Part print with two shaded views. Sizes in mm from the minimum x, y, z corner. A direction names the side the tool comes from. Coordinates: 2 decimals unless noted, no trailing zeros. Loops run counter-clockwise (first coordinate to the right, second up) from the corner with the lowest first, then second, coordinate; pieces in that order, holes last.
(1) Wall check: L1, parallel to Y at x = 14, z = 1.5; L2, parallel to Y at x = 14, z = 6.75; L3, parallel to X at y = 18, z = 1.5 (1 decimal). Give the ranges that are in metal, low to high.
(2) Slice it at C-C (z = 1). Give the cut face in (x, y).
(3) Two-plate mould, pull along Y, no slides. Class the marked faces 1, 2 and 3: pulls with the +Y half, pulls with the -Y half, needs draft (parallel to the pull), parting line crosses it, or undercut.
(4) Slice it at B-B (y = 14). Give the cut face in (x, z), and give its area (3 significant figures).
(5) Tool access for the marked faces 4 and 5: list every direction of +Z, -Z, +X, -X, +Y, -Y with a clear straight run to the whole face (end or side of a thin tool).
(6) Flat gauge pins, fed straight in: P1, Ø1.5, axis at y = 15.5, z = 5, coming from the +X side; P2, Ø2.5, axis at x = 23.09, y = 8.75, coming from the +Z side; P3, Ø8, axis at x = 14, y = 14, coming from the +Z side; P4, Ø1.5, axis at y = 10.5, z = 7.5, coming from the +X side. Where does each tip first touch, or does it go through?
(7) Slice it at D-D (z = 8.5). Give the cut face in (x, y), and give its area (3 significant figures).
(8) Slice it at A-A (x = 14). Give the cut face in (y, z).
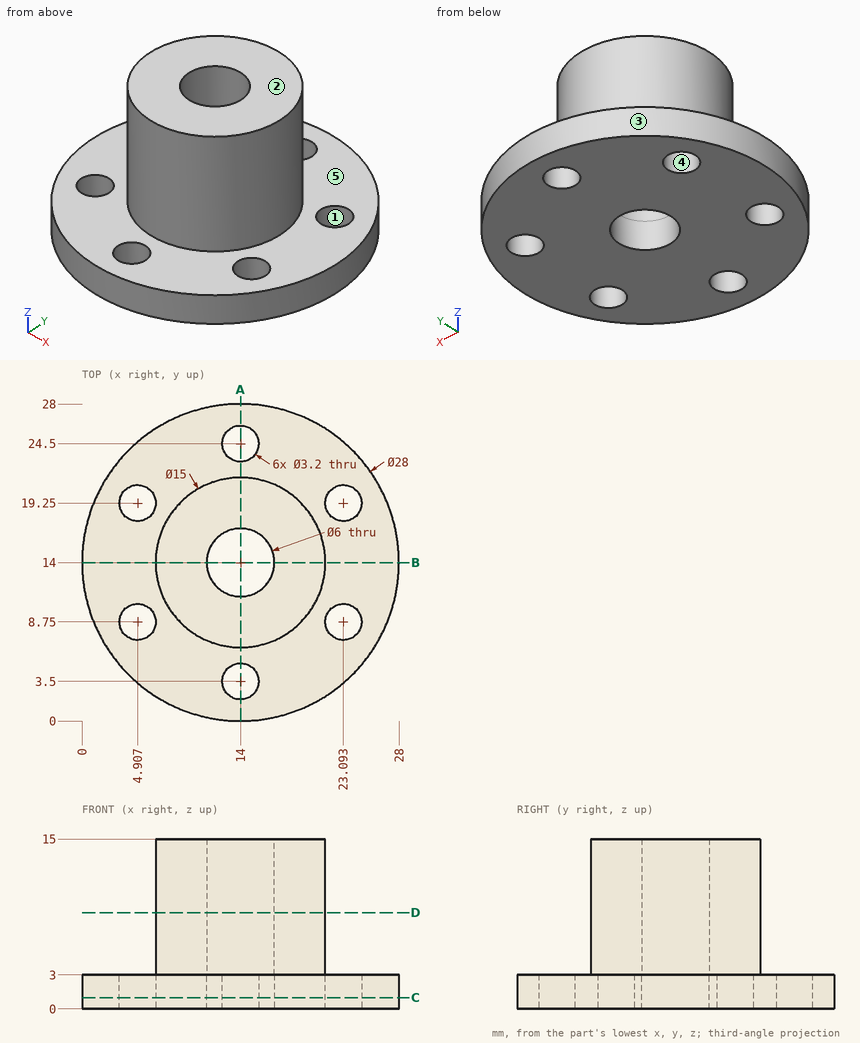
Response values:
1. L1: y = 0 to 1.9, 5.1 to 11, 17 to 22.9, 26.1 to 28
1. L2: y = 6.5 to 11, 17 to 21.5
1. L3: x = 0.6 to 3.9, 5.9 to 22.1, 24.1 to 27.4
2. outline: circle Ø28 at (14, 14); hole circle Ø3.2 at (4.91, 8.75); hole circle Ø3.2 at (4.91, 19.25); hole circle Ø6 at (14, 14); hole circle Ø3.2 at (14, 3.5); hole circle Ø3.2 at (14, 24.5); hole circle Ø3.2 at (23.09, 8.75); hole circle Ø3.2 at (23.09, 19.25)
3. face 1: undercut
3. face 2: needs draft
3. face 3: parting line crosses it
4. outline: (0, 0) - (11, 0) - (11, 15) - (6.5, 15) - (6.5, 3) - (0, 3) - close; (17, 0) - (28, 0) - (28, 3) - (21.5, 3) - (21.5, 15) - (17, 15) - close
4. area: 174 mm2
5. face 4: +Z, -Z
5. face 5: +Z
6. P1: stops at x = 21.46
6. P2: passes through
6. P3: stops at z = 15
6. P4: stops at x = 20.98
7. outline: circle Ø15 at (14, 14); hole circle Ø6 at (14, 14)
7. area: 148 mm2
8. outline: (0, 0) - (1.9, 0) - (1.9, 3) - (0, 3) - close; (5.1, 0) - (11, 0) - (11, 15) - (6.5, 15) - (6.5, 3) - (5.1, 3) - close; (17, 0) - (22.9, 0) - (22.9, 3) - (21.5, 3) - (21.5, 15) - (17, 15) - close; (26.1, 0) - (28, 0) - (28, 3) - (26.1, 3) - close
